Solid Edge part; units mm, degrees
sketch "Sketch1" plane through (0, 0, 0) normal (1, 0, 0) x (0, 1, 0)
  line L0 (-10, -40) -> (10, -40)
  line L1 (10, -40) -> (10, 40)
  line L2 (10, 40) -> (-10, 40)
  line L3 (-10, 40) -> (-10, -40)
  dimension "D1" = 10
  dimension "D2" = 10
extrude "Protrusion1" add sketch "Sketch1" along normal blind 175
sketch "Sketch2" plane through (61, -10, 0) normal (0, -1, 0) x (1, 0, 0)
  circle A0 centre (81.5, 17) radius 6
extrude "Cutout1" cut sketch "Sketch2" against normal through all and the other way through all
sketch "Sketch3" plane through (0, 0, 0) normal (-1, 0, 0) x (0, -1, 0)
  arc A0 (5, -25) -> (-10, -40) centre (-10, -25) cw
  line L0 (5, 25) -> (5, -25)
  arc A1 (5, 25) -> (-10, 40) centre (-10, 25) ccw
  dimension "D1" = 5
extrude "Cutout2" cut sketch "Sketch3" against normal through all material side at (0, -0.642, -35.642)
sketch "Sketch4" plane through (0, 2.399, 0) normal (-1, 0, 0) x (0, 0, 1)
  line L0 (-5, -4.899) -> (5, -4.899)
  line L1 (5, -4.899) -> (5, 5.101)
  line L2 (5, 5.101) -> (-5, 5.101)
  line L3 (-5, 5.101) -> (-5, -4.899)
  dimension "D1" = 5
extrude "Extrusionsausprägung_3" add sketch "Sketch4" along normal blind 25
sketch "Sketch5" plane through (86, 10, 0) normal (0, 1, 0) x (-1, 0, 0)
  circle A0 centre (36, 15.63) radius 1.875
  circle A1 centre (-19, 15.63) radius 1.875
  dimension "D1" = 36
extrude "Cutout3" cut sketch "Sketch5" against normal through all
chamfer "Fase_1" distance 0.7 angle 60 3 edges at (106.875, 10, 15.63) (142.5, 10, 23) (51.875, 10, 15.63) measured on face at (144.0833, 10, -27.4667)
mirror "Mirror1" about plane through (0, 0, 0) normal (0, 0, 1) of "Cutout1", "Cutout3"
properties part number "C1.1-A" material "Nylon, allgemein"
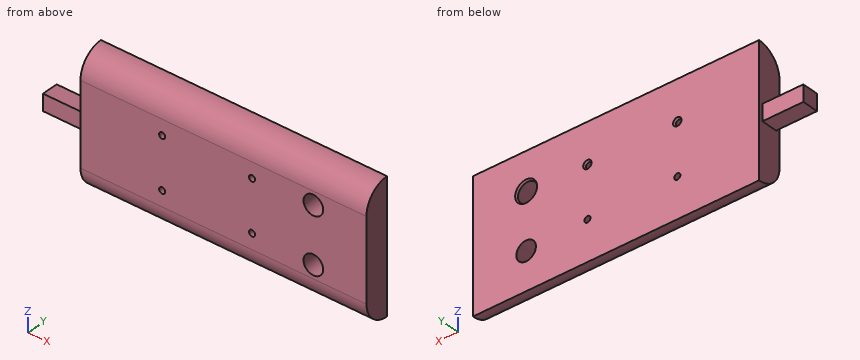
Here's how the part is built. I have some questions about the finished solid (model axes, mm). Give positions to 0.01 mm unless a question says otherwise; leave off trailing zeros. Write each loop counter-clockwise with the first axis right and the second up, starting at its lowest first coordinate (ties: lowest second). Pieces come first, ordered by that corner, then holes. Notation, with made-up numbers: (-2, 65) -> (18, 65) arc R29 ccw to (18, 86) -> close; hole circle Ø9 at (16, 51). An arc over 180 degrees is marked (long way). Use one line per item in the form item = value. Start each with the question number.
1. Imagine slicing it at A-A on x = 50. List the corners of the cut face in (y, z) for me (3 decimals).
2. Imagine slicing it at C-C on y = 5.75. List the corners of the cut face in (x, z) for me (3 decimals).
3. Imagine slicing it at D-D on z = -8.5. List the corners of the cut face in (x, y) for me.
4. If I drill on L1, parallel to Z at x = 105, y = -0.5 (3 decimals); L2, parallel to Z at x = 50, y = 6 (3 decimals); L3, parallel to X at y = 4.25, z = -15.63 (1 decimal), over which ranges is the centre line in solid material (lowest first)?
5. Will these pins go through, and if not, where does the flat tip stop? pin 1 Ø3 at (x, z) = (-18.5, 2.5) entering from +Y; pin 2 Ø4.5 at (x, z) = (105, 15.63) entering from +Y; pin 3 Ø2 at (y, z) = (2, -15) entering from -X.
6. Imagine slicing it at B-B on z = -19.5. List the corners of the cut face in (x, y) for me.
Entries:
q1.outline = (-5, -25) arc R15 ccw to (10, -40) -> (10, -17.505) -> (-5, -17.505) -> close; (-5, -13.755) -> (10, -13.755) -> (10, 13.055) -> (8.788, 13.755) -> (-5, 13.755) -> close; (-5, 17.505) -> (8.788, 17.505) -> (10, 18.205) -> (10, 40) arc R15 ccw to (-5, 25) -> close
q2.outline = (-25, -5) -> (0, -5) -> (0, -39.385) -> (175, -39.385) -> (175, 39.385) -> (0, 39.385) -> (0, 5) -> (-25, 5) -> close; hole circle Ø3.75 at (50, -15.63); hole circle Ø3.75 at (50, 15.63); hole circle Ø3.75 at (105, -15.63); hole circle Ø3.75 at (105, 15.63); hole circle Ø12 at (142.5, -17); hole circle Ø12 at (142.5, 17)
q3.outline = (0, -5) -> (175, -5) -> (175, 10) -> (0, 10) -> close
q4.L1 = -35.712 to -17.505, -13.755 to 13.755, 17.505 to 35.712
q4.L2 = -39.457 to -17.505, -13.755 to 13.755, 17.505 to 39.457
q4.L3 = 0 to 48.1, 51.9 to 103.1, 106.9 to 136.7, 148.3 to 175
q5.pin_1 = 7.5
q5.pin_2 = 9.44
q5.pin_3 = 0
q6.outline = (0, -5) -> (137.05, -5) -> (137.05, 10) -> (0, 10) -> close; (147.95, -5) -> (175, -5) -> (175, 10) -> (147.95, 10) -> close
